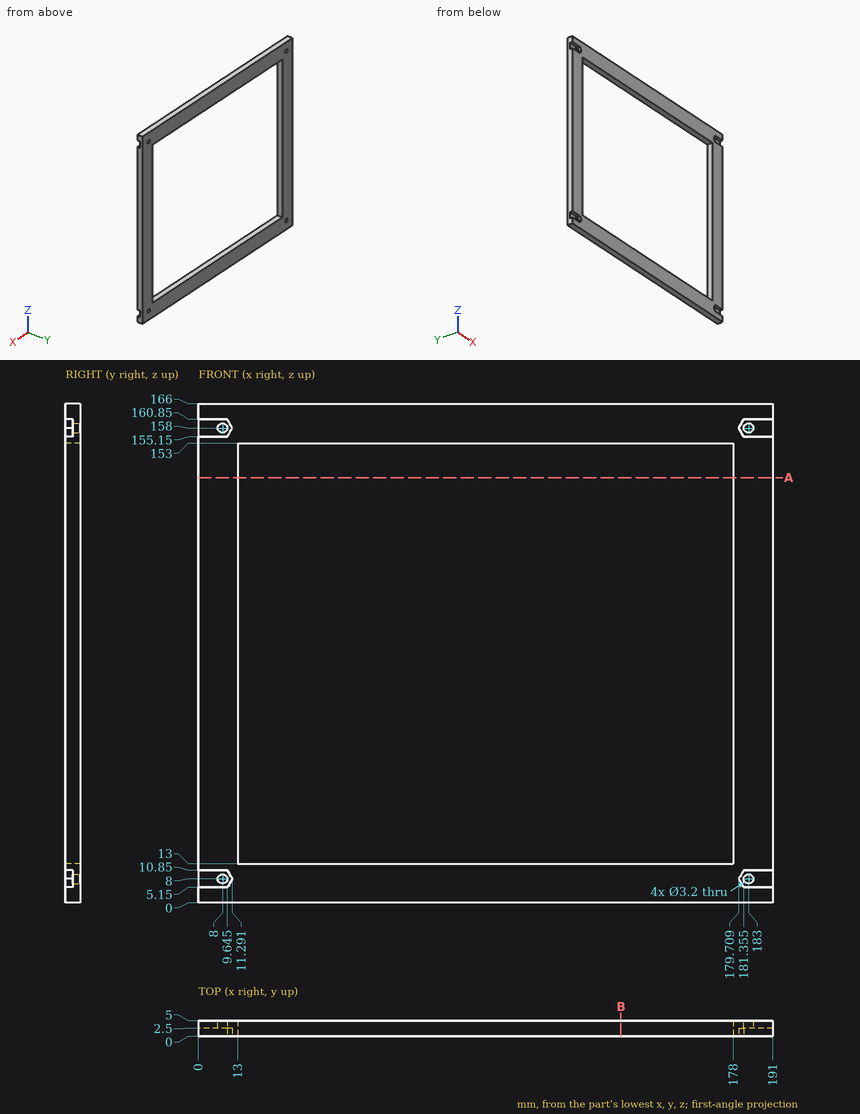
Source: three-view drawing plus pictorial views. Frame: mm from the lowest corner of the part. Round coordinates to 2 decimals unless told otherwise and drop trailing zeros. Loops run counter-clockwise (first coordinate to the right, second up) from the corner with the lowest first, then second, coordinate; pieces in that order, holes last.
Q1. Material intervals for L1, parallel to Z at x = 183, y = 4; L2, parallel to X at y = 3.2, z = 8; L3, parallel to X at y = 0.3, z = 26.5, sorted ascending.
Q2. Section B-B on x = 140.5. Return loops of the section in (y, z), plus the area to 3 significant figures.
Q3. Pin query (flat end, axial travel): P1, Ø1.7, axis at x = 186, z = 158.5, coming from the -Y side. Return the tip coordinate at first contact, or that it passes through.
Q4. Section A-A on z = 141.5. Return loops of the section in (x, y), plus the area to 3 significant figures.
Evaluation:
1. L1: z = 0 to 6.4, 9.6 to 156.4, 159.6 to 166
1. L2: x = 0 to 6.4, 9.6 to 181.4, 184.6 to 191
1. L3: x = 0 to 13, 178 to 191
2. outline: (0, 0) - (5, 0) - (5, 13) - (0, 13) - close; (0, 153) - (5, 153) - (5, 166) - (0, 166) - close
2. area: 130 mm2
3. P1: stops at y = 2.5
4. outline: (0, 0) - (13, 0) - (13, 5) - (0, 5) - close; (178, 0) - (191, 0) - (191, 5) - (178, 5) - close
4. area: 130 mm2
